```python
from build123d import *

# Parameters (mm, degrees)
BASE_EXTRUDE_DEPTH = 101.6
HOLE1_START        = -8.7122
HOLE1_OUTLINE_R    = 7.14375
HOLE1_DEPTH        = 1.4986
LPATTERN2_COUNT    = 2
LPATTERN2_PITCH    = 47.625


# Read off the part's stored shape, not the designer's step: Hole1
with BuildPart() as part:
    # Sketch1 → Base-Extrude (new body)
    with BuildSketch(Plane.XY):
        with BuildLine():
            Line((-20.6375, 10.4394), (-20.6375, 2.59565134))
            ThreePointArc((-20.6375, 2.59565134), (-19.1389, 0), (-20.6375, -2.59565134))
            Line((-20.6375, -2.59565134), (-20.6375, -7.2136))
            ThreePointArc((-20.6375, -7.2136), (-20.198570222, -8.273270222), (-19.1389, -8.7122))
            Line((-19.1389, -8.7122), (19.1389, -8.7122))
            ThreePointArc((19.1389, -8.7122), (20.198570222, -8.273270222), (20.6375, -7.2136))
            Line((20.6375, -7.2136), (20.6375, -2.59565134))
            ThreePointArc((20.6375, -2.59565134), (19.1389, 0), (20.6375, 2.59565134))
            Line((20.6375, 2.59565134), (20.6375, 10.4394))
            ThreePointArc((20.6375, 10.4394), (20.198570222, 11.499070222), (19.1389, 11.938))
            Line((19.1389, 11.938), (12.6111, 11.938))
            ThreePointArc((12.6111, 11.938), (11.551429778, 11.499070222), (11.1125, 10.4394))
            Line((11.1125, 10.4394), (11.1125, 5.588))
            Line((11.1125, 5.588), (12.6111, 5.588))
            Line((12.6111, 5.588), (12.6111, 10.4394))
            Line((12.6111, 10.4394), (19.1389, 10.4394))
            Line((19.1389, 10.4394), (19.1389, 3.350971471))
            ThreePointArc((19.1389, 3.350971471), (17.6403, 0), (19.1389, -3.350971471))
            Line((19.1389, -3.350971471), (19.1389, -7.2136))
            Line((19.1389, -7.2136), (-19.1389, -7.2136))
            Line((-19.1389, -7.2136), (-19.1389, -3.350971471))
            ThreePointArc((-19.1389, -3.350971471), (-17.6403, 0), (-19.1389, 3.350971471))
            Line((-19.1389, 3.350971471), (-19.1389, 10.4394))
            Line((-19.1389, 10.4394), (-12.6111, 10.4394))
            Line((-12.6111, 10.4394), (-12.6111, 5.588))
            Line((-12.6111, 5.588), (-11.1125, 5.588))
            Line((-11.1125, 5.588), (-11.1125, 10.4394))
            ThreePointArc((-11.1125, 10.4394), (-11.551429778, 11.499070222), (-12.6111, 11.938))
            Line((-12.6111, 11.938), (-19.1389, 11.938))
            ThreePointArc((-19.1389, 11.938), (-20.198570222, 11.499070222), (-20.6375, 10.4394))
        make_face()
    extrude(amount=BASE_EXTRUDE_DEPTH)

    # Hole1 outline → Hole1 (cut)
    with BuildSketch(Plane(origin=(0, 0, 0), x_dir=(1, 0, 0), z_dir=(0, 1, 0)).offset(HOLE1_START)):
        with Locations((0, -23.8125)):
            Circle(HOLE1_OUTLINE_R)
    hole1 = extrude(amount=HOLE1_DEPTH, mode=Mode.SUBTRACT)

    # LPattern2: Hole1 ×2
    with Locations(*[(0, 0, i * LPATTERN2_PITCH) for i in range(1, LPATTERN2_COUNT)]):
        add(hole1, mode=Mode.SUBTRACT)


solid = part.part
```
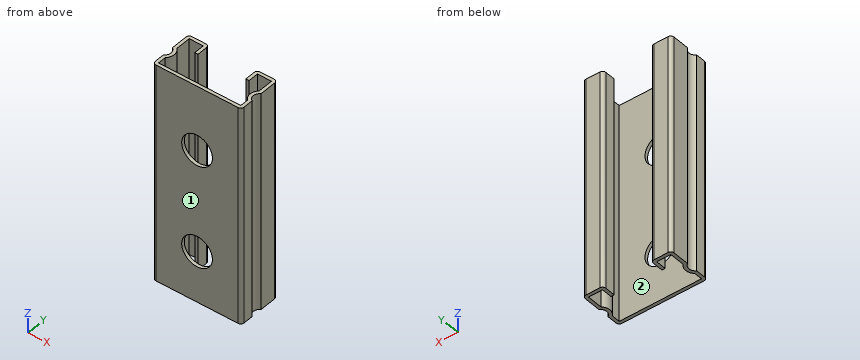
Geometry check sheet. Reference: the model listing, model coordinates, mm. Face numbers are marked on the shaded views. Coordinates: 2 decimals unless noted, no trailing zeros. Order: outer loops, then holes, each group sorted by start corner. A loop starts at its lowest first (then second) coordinate and runs counter-clockwise, first axis right, second up. Notation, with made-up numbers: (-34, 84.25) - (19, 84.25) arc R8 cw to (19, 91.25) - close; hole circle Ø2 at (49.25, 58.5). An arc over 180 degrees is marked (long way). Answer in a Markdown table with one row per item. Add a question column.
1. Section check A-A (y = -5.25). Enter the section's corners in (x, z), plus the area to 3 significant figures.
2. Section check D-D (x = -16.5). Enter the section's corners in (y, z), plus the area to 3 significant figures.
3. Draft check along X on the marked faces 1 and 2. Enter one of: +X half, -X half, draft (parallel to the pull), parting line (faces both ways), or undercut.
4. Section check B-B (x = 0). Enter the section's corners in (y, z), plus the area to 3 significant figures.
5. Gauge pin test, flat ends, axial feed: pin 1 Ø13 at (x, z) = (0, 71.44) entering from -Y; pin 2 Ø2 at (y, z) = (0, 71) entering from -X. Record the tip position at first contact, or that the pin passes through.
6. Material ranges on L1, parallel to X at y = 8.5, z = 97.5; L2, parallel to Z at x = 0, y = -7.8; L3, parallel to X at y = 10.5, z = 63.5, recorded low to high. Write a range as [from, to].
Data:
| question | item | result |
|---|---|---|
| 1 | outline | (-20.64, 0) - (-19.14, 0) - (-19.14, 101.6) - (-20.64, 101.6) - close; (19.14, 0) - (20.64, 0) - (20.64, 101.6) - (19.14, 101.6) - close |
| 1 | area | 305 mm² |
| 2 | outline | (-8.71, 0) - (-7.21, 0) - (-7.21, 101.6) - (-8.71, 101.6) - close; (10.44, 0) - (11.94, 0) - (11.94, 101.6) - (10.44, 101.6) - close |
| 2 | area | 305 mm² |
| 3 | face 1 | draft |
| 3 | face 2 | undercut |
| 4 | outline | (-8.71, 0) - (-7.21, 0) - (-7.21, 16.67) - (-8.71, 16.67) - close; (-8.71, 30.96) - (-7.21, 30.96) - (-7.21, 64.29) - (-8.71, 64.29) - close; (-8.71, 78.58) - (-7.21, 78.58) - (-7.21, 101.6) - (-8.71, 101.6) - close |
| 4 | area | 109 mm² |
| 5 | pin 1 | passes through |
| 5 | pin 2 | stops at x = -19.31 |
| 6 | L1 | x = [-20.64, -19.14], [-12.61, -11.11], [11.11, 12.61], [19.14, 20.64] |
| 6 | L2 | z = [0, 16.67], [30.96, 64.29], [78.58, 101.6] |
| 6 | L3 | x = [-20.64, -11.11], [11.11, 20.64] |
